Read the model definition and answer for the solid it produces. Units are mm, in the model's axes. A direction names the side the tool comes from. Round coordinates to 2 decimals unless told otherwise and drop trailing zeros. Write each loop counter-clockwise with the first axis right and the second up, starting at its lowest first coordinate (ties: lowest second). Pieces come first, ordered by that corner, then holes. Notation, with made-up numbers: (22, 4.5) -> (66, 4.5) arc R12 ccw to (66, 22.5) -> close; hole circle Ø2 at (63, 3). An arc over 180 degrees is marked (long way). Return JSON: item names as keys, results as strings. Group by question number.
(1) Given pin 1 (3 mm diameter, centred on x = 0, z = 6, fed in from +Y); pin 2 (5 mm diameter, centred on x = -12.5, y = -26.5, fed in from -Z); pin 3 (5 mm diameter, centred on x = 12, y = -59, fed in from -Z); pin 4 (6 mm diameter, centred on x = -12.5, z = 15, fed in from -Y), each flat-ended and moving along its own axis, determine where each tip first touches the part or whether it passes through.
(2) For faces 4 (the cylindrical face through (-14.274, -103.165, 0.628)), 5 (the cylindrical face through (1.38, -51.65, -6.2)), 6 (the cylindrical face through (-15.12, -109.82, -11.59)), determine the directions among +Z, -Z, +X, -X, +Y, -Y from which every point of the face is accessible in a straight line to the end or side of a thin tool.
(3) The mould has two halves that part along Y. Classify faces 1 (the flat face through (0, -117.475, 0)), 2 (the flat face through (-5, -101.6, 14)), 3 (the cylindrical face through (-15.12, -50.12, -11.59)): released by +Y, released by -Y, zero draft, split by the parting line, or undercut.
(4) A cutting plane is placed at C-C on y = -34. Give the vertices of the cut face in (x, z).
(5) Straight lines are drawn through the part: line 1 (Z direction, x = 0, y = -32.5); line 2 (Y direction, x = 5.5, z = -16); line 3 (X direction, y = -69, z = -1.5). For each, find the intervals that lie inside material, in ascending order.
```python
from build123d import *

# Parameters (mm, degrees)
F0_R      = 19.05
F1_DEPTH  = 101.6
F2_R      = 2.54
F5_R      = 14.2875
F5_R_2    = 6.35
F6_DEPTH  = 3.175
F7_R      = 19.05
F7_R_2    = 14.2875
F8_DEPTH  = 25.4
F10_R     = 19.05
F11_DEPTH = 12.7
F12_R     = 2.54
F13_R     = 5.08
F3_R      = 6.35
F14_DEPTH = 104.775


# Not quite as in the source:
# - a feature names something its author has since deleted; it is built from what else it names


with BuildPart() as f1:
    # F0 (on Front) → F1 (new body)
    with BuildSketch(Plane.XZ):
        Circle(F0_R)
    extrude(amount=F1_DEPTH)

    # F2
    f2_edges = [f1.edges().sort_by_distance(p)[0] for p in [
        (-19.05, -101.6, 0),
        (-19.05, 0, 0),
    ]]
    fillet(f2_edges, radius=F2_R)

    # F5 (on face) → F6 (join)
    with BuildSketch(Plane.XZ.offset(101.6)):
        Circle(F5_R)
        Circle(F5_R_2, mode=Mode.SUBTRACT)
    extrude(amount=F6_DEPTH)

    # F10 (on face) → F11 (join)
    with BuildSketch(Plane.XZ.offset(104.775)):
        Circle(F10_R)
    extrude(amount=F11_DEPTH)

    # F12
    f12_edges = [f1.edges().sort_by_distance(p)[0] for p in [
        (-19.05, -104.775, 0),
    ]]
    fillet(f12_edges, radius=F12_R)

    # F13
    f13_edges = [f1.edges().sort_by_distance(p)[0] for p in [
        (-19.05, -117.475, 0),
    ]]
    fillet(f13_edges, radius=F13_R)

    # F3 (on face) → F14 (cut, through all)
    with BuildSketch(Plane(origin=(0, 0, 0), x_dir=(-1, 0, 0), z_dir=(0, 1, 0))):
        Circle(F3_R)
    extrude(amount=-F14_DEPTH, mode=Mode.SUBTRACT)


with BuildPart() as f8:
    # F7 (on face) → F8 (new body)
    with BuildSketch(Plane.XZ.offset(104.775)):
        Circle(F7_R)
        Circle(F7_R_2, mode=Mode.SUBTRACT)
    extrude(amount=F8_DEPTH)


solid = f1.part
```
Checks:
{
 "1": {"pin 1": "stops at y = 0", "pin 2": "stops at z = -16.21", "pin 3": "stops at z = -16.51", "pin 4": "stops at y = -116.79"},
 "2": {"face 4": "none", "face 5": "+Y", "face 6": "+Y, -Y"},
 "3": {"face 1": "released by -Y", "face 2": "undercut", "face 3": "zero draft"},
 "4": {"outline": "circle Ø38.1 at (0, 0); hole circle Ø12.7 at (0, 0)"},
 "5": {"line 1": "z = -19.05 to -6.35, 6.35 to 19.05", "line 2": "y = -116.53 to -104.81, -101.57 to -0.03", "line 3": "x = -18.99 to -6.17, 6.17 to 18.99"}
}
